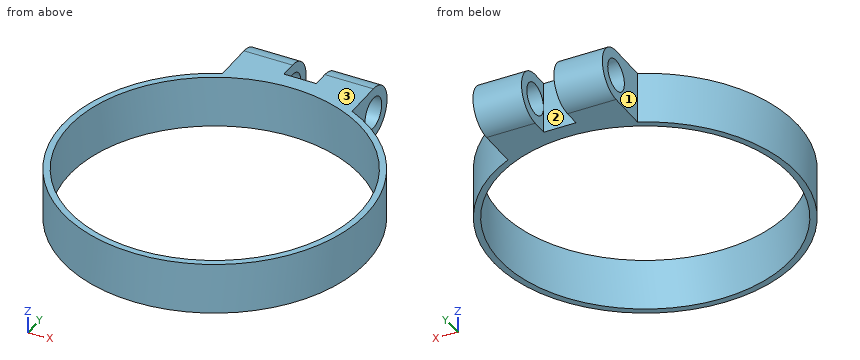
Autodesk Fusion 360 part; units mm, degrees
sketch "Sketch1" plane through (0, 0, 0) normal (0, 0, 1) x (1, 0, 0)
  circle A0 centre (0, 0) radius 45
  circle A1 centre (0, 0) radius 47
  dimension "d1" = 90
  dimension "d3" = 2
extrude "Extrude1" add sketch "Sketch1" along normal blind 16
ref_plane "WorkPlane1" through (55, 0, 0) normal (1, 0, 0) x (0, 1, 0)
sketch "Sketch2" plane through (55, 0, 0) normal (1, 0, 0) x (0, 1, 0)
  circle A0 centre (55, 8) radius 4.875
  circle A1 centre (55, 8) radius 8
  line L0 (47, 16) -> (-47, 16)
  line L1 (47, 0) -> (-47, 0)
  line L2 (47, 16) -> (55, 16)
  line L3 (47, 0) -> (55, 0)
  line L4 (47, 16) -> (42, 16)
  line L5 (42, 16) -> (42, 0)
  line L6 (42, 0) -> (47, 0)
  line L7 (47, 0) -> (47, 16)
  dimension "d7" = 9.75
  dimension "d10" = 5
extrude "Extrude2" add sketch "Sketch2" along normal mid plane 40 from surface at -55
sketch "Sketch3" plane through (0, 0, 16) normal (0, 0, 1) x (-1, 0, 0)
  arc A0 (20, -42.5323) -> (-20, -42.5323) centre (0, 0) ccw
  line L0 (-20, -42.5323) -> (-20, -55)
  line L1 (-20, -55) -> (20, -55)
  line L2 (20, -55) -> (20, -42.5323)
  arc A1 (16.1555, -42) -> (-16.1555, -42) centre (0, 0) ccw
  line L3 (16.1555, -42) -> (-16.1555, -42)
  circle A2 centre (0, 0) radius 45
  line L4 (5, -50) -> (-5, -50)
  line L5 (-5, -50) -> (-5, -65)
  line L6 (-5, -65) -> (5, -65)
  line L7 (5, -65) -> (5, -50)
  dimension "d13" = 5
  dimension "d14" = 5
  dimension "d15" = 50
  dimension "d16" = 15
extrude "Extrude3" cut sketch "Sketch3" against normal through all contours L1 L5 L6 L7 | L1 L4 L5 L7 | A1 L3 A2 | L3 A2
Can you work these out from the model? Positions are in its coordinate system, mm. Face numbers are marked on the shaded views. Coordinates: 2 decimals unless noted, no trailing zeros. Write each loop counter-clockwise with the first axis right and the second up, starting at its lowest first coordinate (ties: lowest second). Pieces come first, ordered by that corner, then holes. Notation, with made-up numbers: (46.5, -24.5) - (101.5, -24.5) arc R34 ccw to (101.5, 13.5) - close; hole circle Ø5 at (83.25, 2). An arc over 180 degrees is marked (long way). Return JSON: item names as keys, results as strings.
Q1. If we section it at D-D (z = 1.25): Please give me the cut outline in (x, y), then the cut area to 3 significant figures.
Computed values:
{"outline": "(-20, 42.53) arc R47 ccw (long way) to (20, 42.53) - (20, 59.29) - (5, 59.29) - (5, 50) - (-5, 50) - (-5, 59.29) - (-20, 59.29) - close; hole circle Ø90 at (0, 0)", "area": "1,040 mm2"}
Q2. I'm going to push flat-ended pins straight in: pin 1 Ø6.5 at (y, z) = (59, 10) entering from +X; pin 2 Ø3 at (y, z) = (-25, 6.5) entering from -X; pin 3 Ø1.5 at (y, z) = (28.5, 10) entering from -X; pin 4 Ø6 at (y, z) = (55, 8) entering from -X. Where does each tip first touch, or does it pass through?
Computed values:
{"pin 1": "stops at x = 20", "pin 2": "stops at x = -40.7", "pin 3": "stops at x = -37.93", "pin 4": "passes through"}
Q3. If we section it at C-C (z = 8): Count the separate pieces of the cut face and the enclosed holes in it, then the cut area to 3 significant figures.
Computed values:
{"separate pieces": "3", "enclosed holes": "1", "area": "854 mm2"}
Q4. If we section it at B-B (y = 0): Please give me the cut outline in (x, z), then the cut area to 3 significant figures.
Computed values:
{"outline": "(-47, 0) - (-45, 0) - (-45, 16) - (-47, 16) - close; (45, 0) - (47, 0) - (47, 16) - (45, 16) - close", "area": "64.0 mm2"}
Q5. Thinking about a two-plate mould opening in X: for the marked faces 1, 2 and 3, which applies, +X half, -X half, draft (parallel to the pull), parting line (faces both ways), or undercut?
Computed values:
{"face 1": "-X half", "face 2": "undercut", "face 3": "draft"}
Q6. Please list where these lines run through material, in increasing order: L1, parallel to Z at x = -9.5, y = 55 (3 decimals); L2, parallel to Y at x = 0, z = 4.75; L3, parallel to Y at x = 10.5, z = 8 (3 decimals). Write a range as from..to.
Computed values:
{"L1": "z = 0..3.125, 12.875..16", "L2": "y = -47..-45, 45..50", "L3": "y = -45.812..-43.758, 43.758..50.125, 59.875..63"}
Q7. If we section it at A-A (x = 0): Please give me the cut outline in (y, z), then the cut area to 3 significant figures.
Computed values:
{"outline": "(-47, 0) - (-45, 0) - (-45, 16) - (-47, 16) - close; (45, 0) - (50, 0) - (50, 16) - (45, 16) - close", "area": "112 mm2"}
